Build history of the part. All positions in model axes, mm. Round coordinates to 2 decimals unless told otherwise and drop trailing zeros. Write each loop counter-clockwise with the first axis right and the second up, starting at its lowest first coordinate (ties: lowest second). Pieces come first, ordered by that corner, then holes. Notation, with made-up numbers: (16, 45) -> (20, 45) arc R12 cw to (20, 65) -> close; hole circle Ø6 at (23, 71). An arc over 180 degrees is marked (long way). Answer in a Markdown table with one row per item. Add a question column.
from build123d import *

# Parameters (mm, degrees)
SKETCH1_R           = 1.5
BOSS_EXTRUDE1_DEPTH = 6


with BuildPart() as part:
    # Sketch1 → Boss-Extrude1 (new body)
    with BuildSketch(Plane(origin=(0, 0, 0), x_dir=(1, 0, 0), z_dir=(0, 1, 0))):
        with BuildLine():
            ThreePointArc((-59.687638113, 12.774374027), (-63.854017455, 7.715818425), (-57.675322321, 5.531458557))
            add(Edge.make_bspline(
                [(-57.675322321, 5.531458557), (-48.450214881, 8.368212133), (-29.885063183, 11.107920581), (-11.319911486, 8.159941585), (-1.979867229, 5.310941391)],
                knots=[0.038744628, 0.038744628, 0.038744628, 0.038744628, 0.5, 0.967002213, 0.967002213, 0.967002213, 0.967002213], degree=3))
            ThreePointArc((-1.979867229, 5.310941391), (3.903752715, 7.914399297), (-0.312361887, 12.774374027))
            add(Edge.make_bspline(
                [(-59.687638113, 12.774374027), (-49.791758742, 15.54092351), (-30, 18.307472992), (-10.208241258, 15.54092351), (-0.312361887, 12.774374027)],
                knots=[0.005206031, 0.005206031, 0.005206031, 0.005206031, 0.5, 0.994793969, 0.994793969, 0.994793969, 0.994793969], degree=3))
        make_face()
        with Locations((-60, 8.786588921)):
            Circle(SKETCH1_R, mode=Mode.SUBTRACT)
        with Locations((0, 8.786588921)):
            Circle(SKETCH1_R, mode=Mode.SUBTRACT)
    extrude(amount=BOSS_EXTRUDE1_DEPTH)


solid = part.part
(1) Drop flat-ended pins along their axis: P1, Ø2.5, axis at x = 0, z = -8.79, coming from the +Y side; P2, Ø1, axis at y = 3, z = -12, coming from the +X side; P3, Ø3, axis at x = -42.5, y = 2.5, coming from the +Z side; P4, Ø2, axis at x = -17, y = 2, coming from the -Z side. Give the stop position or say it passes through.
(2) Saw through at B-B (z = -11). List the corners of the cut face in (x, y).
(3) Saw through at A-A (y = 3.75). Count the separate pieces of the cut face and the enclosed holes in it, plus the area to 3 significant figures.
(4) Mould opens along Z. For faces 1 (the face through (-0.195, 2.958, -10.274)), 2 (the face through (-30, 6, -12)), 3 (the face through (3.88, 2.96, -7.81)) say: pulls with the +Z half, pulls with the -Z half, needs draft (parallel to the pull), parting line crosses it, or undercut.
(5) Probe line 1 along Z through (x, y) = (0, 2.95); line 2 along Z through (x, y) = (-27.5, 1.5); line 3 along Z through (x, y) = (-18.5, 2.25). List the from-to ranges inside material, lowest first.
Answer sheet:
| question | item | result |
|---|---|---|
| 1 | P1 | passes through |
| 1 | P2 | stops at x = 2.94 |
| 1 | P3 | stops at z = -8.66 |
| 1 | P4 | stops at z = -16.25 |
| 2 | outline | (-63.33, 0) -> (3.33, 0) -> (3.33, 6) -> (-63.33, 6) -> close |
| 3 | separate pieces | 1 |
| 3 | enclosed holes | 2 |
| 3 | area | 485 mm² |
| 4 | face 1 | undercut |
| 4 | face 2 | needs draft |
| 4 | face 3 | parting line crosses it |
| 5 | line 1 | z = -12.79 to -10.29, -7.29 to -4.79 |
| 5 | line 2 | z = -16.89 to -9.64 |
| 5 | line 3 | z = -16.3 to -8.91 |
